The model under review builds one solid part; all positions refer to its coordinate system, in mm. A direction names the side the tool comes from. Give positions to 0.01 mm unless a question says otherwise; leave off trailing zeros. Loops run counter-clockwise (first coordinate to the right, second up) from the corner with the lowest first, then second, coordinate; pieces in that order, holes last. Notation, with made-up numbers: M 50.5,46 L 97.5,46 A22 ccw 97.5,85 Z; hole C 77,12 d1. An arc over 180 degrees is marked long. One line per item, written item: value. Start each with the question number.
Q1. For faces 1 (the face through (0.601, 9.754, -97.092)), 2 (the face through (9.5, 0, -122)), list the 3-axis set-ups (+Z, -Z, +X, -X, +Y, -Y) from which the entire face can be reached by the end or side of a thin tool; tool diameter is ignored.
Q2. Mouldability with a two-part tool opening along Y and no side actions: class faces 3 (the face through (-9.5, 0, -122)), 4 (the face through (-2, 10, -122)), 5 (the face through (-2, -10, -122)), 6 (the face through (0.601, -9.747, -72.092)) as released by +Y, released by -Y, zero draft, split by the parting line, or undercut.
Q3. We need section A-A on z = -174. Write out the cut boundary in (x, y), plus the area to 3 significant figures.
Q4. We need section B-B on x = -6.5. Write out the cut boundary in (y, z).
Q5. To check wall thickness, follow line 1 along Y through (x, z) = (7.5, -22); line 2 along X through (y, z) = (9.7, -12.25). State the ranges of each line that lie inside material, in increasing order. Write a range as from..to.
Q6. We need section D-D on z = -34.5. Write out the cut boundary in (x, y).
```python
from build123d import *

# Parameters (mm, degrees)
SKETCH_1_W          = 20
SKETCH_1_H          = 20
SKETCH_1_W_2        = 19
SKETCH_1_H_2        = 19
EXTRUDE_1_DEPTH     = 248
SKETCH_2_R          = 2
CUT_EXTRUDE_1_DEPTH = 250.006024024
SKETCH_3_R          = 2
CUT_EXTRUDE_2_DEPTH = 250.006024024
SKETCH_4_R          = 1.7
CUT_EXTRUDE_3_DEPTH = 250.006024024


with BuildPart() as part:
    # 草图1 → 凸台-拉伸1 (new body)
    with BuildSketch(Plane.XY):
        Rectangle(SKETCH_1_W, SKETCH_1_H)
        Rectangle(SKETCH_1_W_2, SKETCH_1_H_2, mode=Mode.SUBTRACT)
    extrude(amount=-EXTRUDE_1_DEPTH)

    # 草图2 → 切除-拉伸1 (cut, through all)
    with BuildSketch(Plane(origin=(0, 10, 0), x_dir=(1, 0, 0), z_dir=(0, 1, 0))):
        with Locations(Location((4.171407716, 12.25, 0), (0, 0, 270))):
            Circle(SKETCH_2_R)
        with Locations((4.171407716, 235.75)):
            Circle(SKETCH_2_R)
    extrude(amount=-CUT_EXTRUDE_1_DEPTH, mode=Mode.SUBTRACT)

    # 草图3 → 切除-拉伸2 (cut, through all)
    with BuildSketch(Plane(origin=(0, 10, 0), x_dir=(1, 0, 0), z_dir=(0, 1, 0))):
        with Locations(Location((0, 74, 0), (0, 0, 270))):
            Circle(SKETCH_3_R)
        with Locations(Location((0, 99, 0), (0, 0, 270))):
            Circle(SKETCH_3_R)
        with Locations(Location((0, 124, 0), (0, 0, 270))):
            Circle(SKETCH_3_R)
        with Locations(Location((0, 149, 0), (0, 0, 270))):
            Circle(SKETCH_3_R)
        with Locations(Location((0, 174, 0), (0, 0, 270))):
            Circle(SKETCH_3_R)
    extrude(amount=-CUT_EXTRUDE_2_DEPTH, mode=Mode.SUBTRACT)

    # 草图4 → 切除-拉伸3 (cut, through all)
    with BuildSketch(Plane(origin=(10, 0, 0), x_dir=(0, 0, -1), z_dir=(1, 0, 0))):
        with Locations((42, 0)):
            Circle(SKETCH_4_R)
        with Locations((206, 0)):
            Circle(SKETCH_4_R)
    extrude(amount=-CUT_EXTRUDE_3_DEPTH, mode=Mode.SUBTRACT)


solid = part.part
```
Solved:
1. face 1: +Y, -Y
1. face 2: +Z, -Z
2. face 3: undercut
2. face 4: released by +Y
2. face 5: released by -Y
2. face 6: zero draft
3. outline: M -10,-10 L -2,-10 L -2,-9.5 L -9.5,-9.5 L -9.5,9.5 L -2,9.5 L -2,10 L -10,10 Z; M 2,-10 L 10,-10 L 10,10 L 2,10 L 2,9.5 L 9.5,9.5 L 9.5,-9.5 L 2,-9.5 Z
3. area: 35.0 mm2
4. outline: M -10,-248 L -9.5,-248 L -9.5,0 L -10,0 Z; M 9.5,-248 L 10,-248 L 10,0 L 9.5,0 Z
5. line 1: -10..-9.5, 9.5..10
5. line 2: -10..2.17, 6.17..10
6. outline: M -10,-10 L 10,-10 L 10,10 L -10,10 Z; hole M -9.5,-9.5 L 9.5,-9.5 L 9.5,9.5 L -9.5,9.5 Z
